from build123d import *

# Parameters (mm, degrees)
MAIN_FEATURES_SKETCH_W = 36
MAIN_FEATURES_SKETCH_H = 65
MAIN_FEATURES_SKETCH_R = 12.5
BASE_FILTER_DEPTH      = 2.05
LENS_SURROUND_DEPTH    = 3.05
ARM_DEPTH              = 2.5
FILLET1_R              = 0.5
LONG_ARM_START         = 0.2
LONG_ARM_DEPTH         = 2


with BuildPart() as part:
    # main_features_sketch → base_filter (new body)
    with BuildSketch(Plane.XY):
        Rectangle(MAIN_FEATURES_SKETCH_W, MAIN_FEATURES_SKETCH_H)
        Circle(MAIN_FEATURES_SKETCH_R, mode=Mode.SUBTRACT)
    extrude(amount=BASE_FILTER_DEPTH)

    # main_features_sketch<4> → lens_surround (add)
    with BuildSketch(Plane.XY):
        Polygon((-16.1, 10), (-16.1, 0), (-16.1, -17.1), (16.1, -17.1), (16.1, 0), (16.1, 10), (15.6, 10), (15.1, 3), (15.1, 0), (15.1, -15.1), (-15.1, -15.1), (-15.1, 0), (-15.1, 3), (-15.6, 10), align=None)
    extrude(amount=LENS_SURROUND_DEPTH)

    # arm_sketch → arm (add, symmetric)
    with BuildSketch(Plane(origin=(0, 0, 0), x_dir=(0, -1, 0), z_dir=(-1, 0, 0))):
        with BuildLine():
            Line((13.9, 2.549398771), (14.9, 2.549398771))
            add(Edge.make_bspline(
                [(19.1, 3.55), (14.882914348, 3.55), (14.9, 3.386309971), (14.9, 2.549398771)],
                knots=[0, 0, 0, 0, 1, 1, 1, 1], degree=3))
            Line((19.1, 3.55), (19.1, 2.05))
            Line((19.1, 2.05), (24.1, 2.05))
            Line((24.1, 2.05), (24.1, 3.55))
            Line((24.1, 3.55), (24.1, 4.55))
            Line((24.1, 4.55), (19.1, 4.55))
            add(Edge.make_bspline(
                [(19.1, 4.55), (14.0970617, 4.55), (12.9, 4.338647065), (12.9, 3.134725983)],
                knots=[0, 0, 0, 0, 1, 1, 1, 1], degree=3))
            Line((12.9, 3.134725983), (13.9, 2.549398771))
        make_face()
    extrude(amount=ARM_DEPTH, both=True)

    # Fillet1
    fillet1_edges = [part.edges().sort_by_distance(p)[0] for p in [
        (1.25, -12.9, 3.134725983),
        (0, -13.9, 2.549398771),
    ]]
    fillet(fillet1_edges, radius=FILLET1_R)

    # long_arm_sketch → long_arm (add)
    with BuildSketch(Plane(origin=(-15.1, 0, 0), x_dir=(0, 0, -1), z_dir=(1, 0, 0)).offset(LONG_ARM_START)):
        with BuildLine():
            Line((-2.05, -24.1), (-5.05, -24.1))
            Line((-5.05, -24.1), (-5.05, 1.297726723))
            add(Edge.make_bspline(
                [(-5.05, 1.297726723), (-5.05, 2.39434011), (-2.25, 1.5663534), (-2.25, 0.537583105)],
                knots=[0, 0, 0, 0, 1, 1, 1, 1], degree=3))
            Line((-2.25, 0.537583105), (-2.25, -0.537583105))
            add(Edge.make_bspline(
                [(-3.55, -3.211240123), (-3.55, -2.566791116), (-2.25, -1.290352393), (-2.25, -0.537583105)],
                knots=[0, 0, 0, 0, 1, 1, 1, 1], degree=3))
            Line((-3.55, -3.211240123), (-3.55, -19.1))
            Line((-3.55, -19.1), (-2.05, -19.1))
            Line((-2.05, -19.1), (-2.05, -24.1))
        make_face()
    long_arm = extrude(amount=LONG_ARM_DEPTH)

    # Mirror1: long_arm across plane
    add(long_arm.mirror(Plane(origin=(0, 0, 0), x_dir=(0, 0, 1), z_dir=(1, 0, 0))))


solid = part.part
Could you check a few things on this model? Use its own coordinates, in mm. A direction names the side the tool comes from. Coordinates: 2 decimals unless noted, no trailing zeros. Loops run counter-clockwise (first coordinate to the right, second up) from the corner with the lowest first, then second, coordinate; pieces in that order, holes last.
1. We'd pull the mould along X, two halves only. Please class faces 6 (the face through (-2.5, -20, 4)), 7 (the face through (14, -11, 3.55)), 8 (the face through (-18, 0, 1)): released by +X, released by -X, zero draft, split by the parting line, or undercut.
2. For P1, Ø0.8, axis at y = 0, z = 2.5, coming from the -X side; P2, Ø2.5, axis at x = 1, y = -22.5, coming from the +Z side; P3, Ø0.6, axis at x = 14, z = 3.5, coming from the -Y side, each with a flat end and sliding along its axis, tell me the tip position at first contact or that it passes through.
3. I need wall thicknesses on L1, parallel to Y at x = 0, z = 1; L2, parallel to Y at x = -2, z = 2.95; L3, parallel to X at y = -9.5, z = 4.55. Which ranges of each line are inside material? Lowest first, please.
4. Imagine slicing it at A-A (y = -10). Please give me the cut outline in (x, z).
5. Imagine slicing it at C-C (y = 5). Please give me the cut outline in (x, z).
6. Imagine slicing it at D-D (z = 0.8). Please give me the cut outline in (x, y).
7. For faces 1 (the face through (0, -22, 4.55)), 2 (the face through (-14, -11, 3.55)), 3 (the face through (14, -19.1, 3)), 4 (the face through (-14, -12, 5.05)), 5 (the face through (14, -24.1, 4)), which set-ups out of +Z, -Z, +X, -X, +Y, -Y let a thin tool reach every point of the face, with its end or its side?
8. Imagine slicing it at B-B (x = -7). Please give me the cut outline in (y, z), and give its area (3 significant figures).
Computed values:
1. face 6: undercut
1. face 7: zero draft
1. face 8: released by -X
2. P1: stops at x = -16.1
2. P2: stops at z = 4.55
2. P3: stops at y = -24.1
3. L1: y = -32.5 to -12.5, 12.5 to 32.5
3. L2: y = -24.1 to -19.1, -17.1 to -15.1, -14.93 to -13.22
3. L3: x = -14.9 to -12.9, 12.9 to 14.9
4. outline: (-18, 0) - (-7.5, 0) - (-7.5, 2.05) - (-15.1, 2.05) - (-15.1, 3.05) - (-16.1, 3.05) - (-16.1, 2.05) - (-18, 2.05) - close; (-14.9, 3.55) - (-12.9, 3.55) - (-12.9, 5.05) - (-14.9, 5.05) - close; (7.5, 0) - (18, 0) - (18, 2.05) - (16.1, 2.05) - (16.1, 3.05) - (15.1, 3.05) - (15.1, 2.05) - (7.5, 2.05) - close; (12.9, 3.55) - (14.9, 3.55) - (14.9, 5.05) - (12.9, 5.05) - close
5. outline: (-18, 0) - (-11.46, 0) - (-11.46, 2.05) - (-15.24, 2.05) - (-15.24, 3.05) - (-16.1, 3.05) - (-16.1, 2.05) - (-18, 2.05) - close; (11.46, 0) - (18, 0) - (18, 2.05) - (16.1, 2.05) - (16.1, 3.05) - (15.24, 3.05) - (15.24, 2.05) - (11.46, 2.05) - close
6. outline: (-18, -32.5) - (18, -32.5) - (18, 32.5) - (-18, 32.5) - close; hole circle Ø25 at (0, 0)
7. face 1: +Z, +Y, -Y
7. face 2: -X
7. face 3: +X, -X
7. face 4: +Z, +X, -X, +Y, -Y
7. face 5: +Z, +X, -X, -Y
8. outline: (-32.5, 0) - (-10.36, 0) - (-10.36, 2.05) - (-15.1, 2.05) - (-15.1, 3.05) - (-17.1, 3.05) - (-17.1, 2.05) - (-32.5, 2.05) - close; (10.36, 0) - (32.5, 0) - (32.5, 2.05) - (10.36, 2.05) - close
8. area: 92.8 mm2
